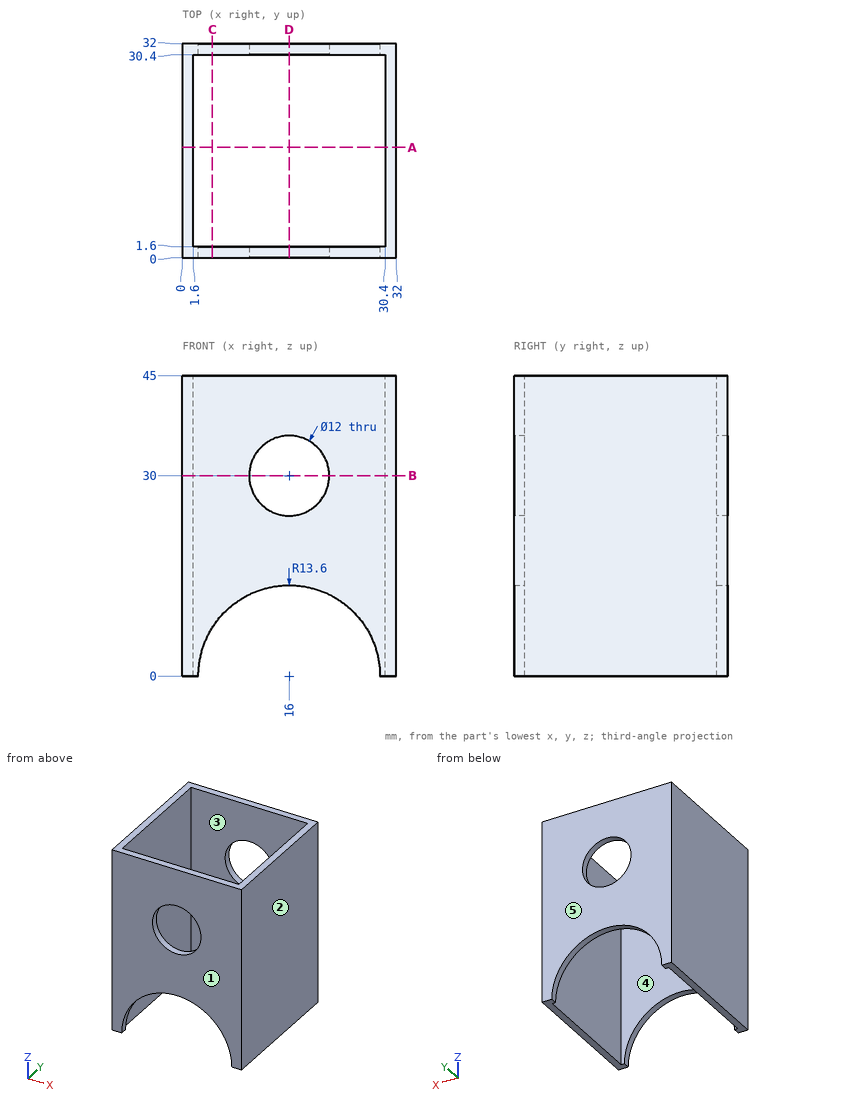
Part print with two shaded views. Sizes in mm from the minimum x, y, z corner. A direction names the side the tool comes from. Round coordinates to 2 decimals unless told otherwise and drop trailing zeros. Order: outer loops, then holes, each group sorted by start corner. A loop starts at its lowest first (then second) coordinate and runs counter-clockwise, first axis right, second up. Notation, with made-up numbers: (57.5, -26) -> (95.5, -26) arc R27 ccw to (95.5, 3) -> close; hole circle Ø9 at (61, -33.5). An arc over 180 degrees is marked (long way). One line per question, with ' | ' between items.
Q1. Slice it at A-A (y = 16.5). Write the cut outline in (x, z), then the cut area to 3 significant figures.
Completed:
outline: (0, 0) -> (1.6, 0) -> (1.6, 45) -> (0, 45) -> close; (30.4, 0) -> (32, 0) -> (32, 45) -> (30.4, 45) -> close | area: 144 mm^2
Q2. Which spindle directions (+Z, -Z, +X, -X, +Y, -Y) get a long thin tool onto all of the face, cutting with end or side? Do the marked faces 4 and 5. Say none if no direction does.
Completed:
face 4: +Z, -Z | face 5: +Z, -Z, +X, -X, +Y
Q3. Slice it at B-B (z = 30). Write the cut outline in (x, y), then the cut area to 3 significant figures.
Completed:
outline: (0, 0) -> (10, 0) -> (10, 1.6) -> (1.6, 1.6) -> (1.6, 30.4) -> (10, 30.4) -> (10, 32) -> (0, 32) -> close; (22, 0) -> (32, 0) -> (32, 32) -> (22, 32) -> (22, 30.4) -> (30.4, 30.4) -> (30.4, 1.6) -> (22, 1.6) -> close | area: 156 mm^2
Q4. Two-plate mould, pull along X, no slides. Class the marked faces 1, 2 and 3: released by +X, released by -X, zero draft, split by the parting line, or undercut.
Completed:
face 1: zero draft | face 2: released by +X | face 3: undercut
Q5. Slice it at C-C (x = 4.5). Write the cut outline in (y, z).
Completed:
outline: (0, 7.26) -> (1.6, 7.26) -> (1.6, 45) -> (0, 45) -> close; (30.4, 7.26) -> (32, 7.26) -> (32, 45) -> (30.4, 45) -> close
Q6. Probe probe 1 along Z at (x, y) = (16, 31.4); probe 2 along X at (y, z) = (17, 37). List the from-to ranges inside material, lowest first.
Completed:
probe 1: z = 13.6 to 24, 36 to 45 | probe 2: x = 0 to 1.6, 30.4 to 32
Q7. Slice it at D-D (x = 16). Write the cut outline in (y, z).
Completed:
outline: (0, 13.6) -> (1.6, 13.6) -> (1.6, 24) -> (0, 24) -> close; (0, 36) -> (1.6, 36) -> (1.6, 45) -> (0, 45) -> close; (30.4, 13.6) -> (32, 13.6) -> (32, 24) -> (30.4, 24) -> close; (30.4, 36) -> (32, 36) -> (32, 45) -> (30.4, 45) -> close
